Autodesk Inventor part; units mm, degrees
ref_plane "YZ Plane" through (0, 0, 0) normal (1, 0, 0) x (0, 1, 0)
ref_plane "XZ Plane" through (0, 0, 0) normal (0, 1, 0) x (-1, 0, 0)
ref_plane "XY Plane" through (0, 0, 0) normal (0, 0, 1) x (1, 0, 0)
sketch "Sketch1" plane through (0, 0, 0) normal (0, 1, 0) x (-1, 0, 0)
  circle A0 centre (0, 0) radius 10
  dimension "d0" = 20
extrude "Extrusion1" add sketch "Sketch1" along normal mid plane 10
sketch "Sketch2" plane through (0, 5, 0) normal (0, 1, 0) x (1, 0, 0)
  circle A0 centre (0, 0) radius 21
  dimension "d3" = 42
extrude "Extrusion2" add sketch "Sketch2" along normal blind 3
sketch "Sketch3" plane through (0, -5, 0) normal (0, -1, 0) x (1, 0, 0)
  circle A0 centre (0, 0) radius 21
  dimension "d6" = 42
extrude "Extrusion3" add sketch "Sketch3" along normal blind 3
sketch "Sketch4" plane through (0, 8, 0) normal (0, 1, 0) x (1, 0, 0)
  circle A0 centre (0, 0) radius 6
  dimension "d9" = 12
extrude "Extrusion4" cut sketch "Sketch4" against normal blind 16
sketch "Sketch7" plane through (0, 8, 0) normal (0, 1, 0) x (1, 0, 0)
  circle A0 centre (0, -16) radius 2.5
  point P0 (0, 0)
  dimension "d13" = 5
extrude "Extrusion5" cut sketch "Sketch7" against normal blind 16
pattern_circular "Circular Pattern1" count 6 over 360 about axis through (0, 5, 0) along (0, 1, 0) of "Extrusion5"
chamfer "Chamfer1" distance 0.5 distance2 0.5 1 edges at (-21, 8, 0) measured on face at (-5.5882, 8, 9.3573)
chamfer "Chamfer2" distance 0.5 distance2 0.5 1 edges at (-21, -8, 0) measured on face at (5.5882, -8, -9.3573)
properties part number "connecting rod hub"
Design review of the part built by this model. Coordinates are the model's own, in mm. Round coordinates to 2 decimals unless told otherwise and drop trailing zeros. Write each loop counter-clockwise with the first axis right and the second up, starting at its lowest first coordinate (ties: lowest second). Pieces come first, ordered by that corner, then holes. Notation, with made-up numbers: (82, -3) - (107, -3) arc R11 ccw to (107, 2) - close; hole circle Ø8 at (26, -38.5). An arc over 180 degrees is marked (long way). Use a Markdown table: item, result. Add a question column.
1. Clearance check with flat-ended pins moving along their axes: pin 1 (2 mm diameter, centred on x = 6.5, y = -3, fed in from +Z); pin 2 (1 mm diameter, centred on y = 1.5, z = -3, fed in from +X); pin 3 (4 mm diameter, centred on y = -3.5, z = -6, fed in from -X). State where each tip first meets the part, or that it passes through.
2. Mouldability with a two-part tool opening along Z and no side actions: class faces 1 (the face through (2.17, 0.07, -9.76)), 2 (the face through (9, 5, -5)), 3 (the face through (-15.84, -6.48, -6.48)) as +Z half, -Z half, draft (parallel to the pull), parting line (faces both ways), or undercut.
3. We need section B-B (y = 6.5). State the section outline as (x, z) points, then the cut area to 3 significant figures.
4. We need section A-A (z = 0). State the section outline as (x, y) points, then the cut area to 4 significant figures.
5. We need section D-D (y = -4.25). State the section outline as (x, z) points, then the cut area to 3 significant figures.
6. Wall thickness on probe 1 along Z at (x, y) = (0, 7.4); probe 2 along Y at (x, z) = (-17.5, 0); probe 3 along Z at (x, y) = (-14, -6): over which ranges is each line inside the solid? List them lowest first.
7. We need section C-C (x = 0). Count the separate pieces of the cut face and the enclosed holes in it, then the cut area to 4 significant figures.
Output:
| question | item | result |
|---|---|---|
| 1 | pin 1 | stops at z = 8.35 |
| 1 | pin 2 | stops at x = 9.68 |
| 1 | pin 3 | stops at x = -20.47 |
| 2 | face 1 | parting line |
| 2 | face 2 | draft |
| 2 | face 3 | undercut |
| 3 | outline | circle Ø42 at (0, 0); hole circle Ø5 at (-13.86, -8); hole circle Ø5 at (-13.86, 8); hole circle Ø12 at (0, 0); hole circle Ø5 at (0, -16); hole circle Ø5 at (0, 16); hole circle Ø5 at (13.86, -8); hole circle Ø5 at (13.86, 8) |
| 3 | area | 1,150 mm2 |
| 4 | outline | (-21, -7.5) - (-20.5, -8) - (-6, -8) - (-6, 8) - (-20.5, 8) - (-21, 7.5) - (-21, 5) - (-10, 5) - (-10, -5) - (-21, -5) - close; (6, -8) - (20.5, -8) - (21, -7.5) - (21, -5) - (10, -5) - (10, 5) - (21, 5) - (21, 7.5) - (20.5, 8) - (6, 8) - close |
| 4 | area | 259.5 mm2 |
| 5 | outline | circle Ø20 at (0, 0); hole circle Ø12 at (0, 0) |
| 5 | area | 201 mm2 |
| 6 | probe 1 | z = -21 to -18.5, -13.5 to -6, 6 to 13.5, 18.5 to 21 |
| 6 | probe 2 | y = -8 to -5, 5 to 8 |
| 6 | probe 3 | z = -15.65 to -10.5, -5.5 to 5.5, 10.5 to 15.65 |
| 7 | separate pieces | 6 |
| 7 | enclosed holes | 0 |
| 7 | area | 199.5 mm2 |
